Read the model definition and answer for the solid it produces. Units are mm, in the model's axes. A direction names the side the tool comes from. Give positions to 0.01 mm unless a question says otherwise; leave off trailing zeros. Write each loop counter-clockwise with the first axis right and the second up, starting at its lowest first coordinate (ties: lowest second). Pieces come first, ordered by that corner, then holes. Notation, with made-up numbers: (29.25, -19.75) - (52.25, -19.75) arc R8 cw to (52.25, -9.75) - close; hole circle Ø9 at (-30.75, -13.75). An arc over 180 degrees is marked (long way). Answer as CSV lines item,"result".
```python
from build123d import *

# Parameters (mm, degrees)
RESSALTO_EXTRUS_O1_DEPTH = 5
FILETE1_R                = 5
ESBO_O3_R                = 1.5
CORTE_EXTRUS_O1_DEPTH    = 5


with BuildPart() as part:
    # Esboço1 → Ressalto-extrusão1 (new body)
    with BuildSketch(Plane(origin=(0, 0, 0), x_dir=(1, 0, 0), z_dir=(0, 1, 0))):
        with BuildLine():
            Line((81.90590785, -20.429188404), (85.90590785, -20.429188404))
            Line((85.90590785, -20.429188404), (85.90590785, 4.570811596))
            ThreePointArc((85.90590785, 4.570811596), (84.441441756, 8.106345502), (80.90590785, 9.570811596))
            Line((80.90590785, 9.570811596), (-32.09409215, 9.570811596))
            ThreePointArc((-32.09409215, 9.570811596), (-35.629626056, 8.106345502), (-37.09409215, 4.570811596))
            Line((-37.09409215, 4.570811596), (-37.09409215, -20.429188404))
            Line((-37.09409215, -20.429188404), (-33.09409215, -20.429188404))
            Line((-33.09409215, -20.429188404), (-33.09409215, -75.429188404))
            Line((-33.09409215, -75.429188404), (-37.09409215, -75.429188404))
            Line((-37.09409215, -75.429188404), (-37.09409215, -100.429188404))
            ThreePointArc((-37.09409215, -100.429188404), (-35.629626056, -103.96472231), (-32.09409215, -105.429188404))
            Line((-32.09409215, -105.429188404), (80.90590785, -105.429188404))
            ThreePointArc((80.90590785, -105.429188404), (84.441441756, -103.96472231), (85.90590785, -100.429188404))
            Line((85.90590785, -100.429188404), (85.90590785, -75.429188404))
            Line((85.90590785, -75.429188404), (81.90590785, -75.429188404))
            Line((81.90590785, -75.429188404), (81.90590785, -20.429188404))
        make_face()
    extrude(amount=RESSALTO_EXTRUS_O1_DEPTH)

    # Filete1
    # the kernel refuses this fillet: 5 mm, written as the material it takes off along each edge
    with BuildSketch(Plane(origin=(-37.09409215, -12.247448714, 75.429188404), x_dir=(1.0, 0, 1.5738521597081158e-12), z_dir=(0, 1, 0)), Plane(origin=(85.90590785, -12.247448714, 20.429188404), x_dir=(-1.0, 0, -1.5685230891899197e-12), z_dir=(0, 1, 0))) as filete1_piece_1:
        with BuildLine():
            CenterArc((5, -4.898979486), FILETE1_R, 101.536959033, 78.463040967)
            Line((0, -4.898979486), (-0.1, -4.898979486))
            Line((-0.1, -4.898979486), (-0.1, 0))
            Line((-0.1, 0), (0, 0.1))
            ThreePointArc((0, 0.1), (2, 0.1), (3.98, 0.09797959))
            Line((3.98, 0.09797959), (4, 0))
        make_face()
    extrude(amount=29.494897428, mode=Mode.SUBTRACT)
    with BuildSketch(Plane(origin=(-37.09409215, -12.247448714, 20.429188404), x_dir=(0, 0, -1), z_dir=(0, 1, 0)), Plane(origin=(85.90590785, -12.247448714, 75.429188404), x_dir=(0, 0, 1), z_dir=(0, 1, 0))) as filete1_piece_2:
        with BuildLine():
            CenterArc((4.898979486, -5), FILETE1_R, 90, 78.463040967)
            Line((0, -4), (-0.09797959, -3.98))
            ThreePointArc((-0.09797959, -3.98), (-0.1, -2), (-0.1, 0))
            Line((-0.1, 0), (0, 0.1))
            Line((0, 0.1), (4.898979486, 0.1))
            Line((4.898979486, 0.1), (4.898979486, 0))
        make_face()
    extrude(amount=29.494897428, mode=Mode.SUBTRACT)

    # Esboço3 → Corte-extrusão1 (cut)
    with BuildSketch(Plane.XZ):
        with Locations(Location((-27.09409215, 5.429188404, 0), (0, 0, 270))):
            Circle(ESBO_O3_R)
        with Locations(Location((75.90590785, 5.429188404, 0), (0, 0, 270))):
            Circle(ESBO_O3_R)
        with Locations(Location((75.90590785, 90.429188404, 0), (0, 0, 90))):
            Circle(ESBO_O3_R)
        with Locations(Location((-27.09409215, 90.429188404, 0), (0, 0, 90))):
            Circle(ESBO_O3_R)
        with BuildLine():
            Line((35.90590785, 84.429188404), (35.90590785, 96.429188404))
            ThreePointArc((35.90590785, 96.429188404), (35.320121412, 97.843401966), (33.90590785, 98.429188404))
            Line((33.90590785, 98.429188404), (31.90590785, 98.429188404))
            ThreePointArc((31.90590785, 98.429188404), (30.491694287, 97.843401966), (29.90590785, 96.429188404))
            Line((29.90590785, 96.429188404), (29.90590785, 84.429188404))
            ThreePointArc((29.90590785, 84.429188404), (30.491694287, 83.014974841), (31.90590785, 82.429188404))
            Line((31.90590785, 82.429188404), (33.90590785, 82.429188404))
            ThreePointArc((33.90590785, 82.429188404), (35.320121412, 83.014974841), (35.90590785, 84.429188404))
        make_face()
        with BuildLine():
            Line((14.90590785, 13.429188404), (16.90590785, 13.429188404))
            ThreePointArc((16.90590785, 13.429188404), (18.320121412, 12.843401966), (18.90590785, 11.429188404))
            Line((18.90590785, 11.429188404), (18.90590785, -0.570811596))
            ThreePointArc((18.90590785, -0.570811596), (18.320121412, -1.985025159), (16.90590785, -2.570811596))
            Line((16.90590785, -2.570811596), (14.90590785, -2.570811596))
            ThreePointArc((14.90590785, -2.570811596), (13.491694287, -1.985025159), (12.90590785, -0.570811596))
            Line((12.90590785, -0.570811596), (12.90590785, 11.429188404))
            ThreePointArc((12.90590785, 11.429188404), (13.491694287, 12.843401966), (14.90590785, 13.429188404))
        make_face()
        with BuildLine():
            Line((23.40590785, 13.429188404), (25.40590785, 13.429188404))
            ThreePointArc((25.40590785, 13.429188404), (26.820121412, 12.843401966), (27.40590785, 11.429188404))
            Line((27.40590785, 11.429188404), (27.40590785, -0.570811596))
            ThreePointArc((27.40590785, -0.570811596), (26.820121412, -1.985025159), (25.40590785, -2.570811596))
            Line((25.40590785, -2.570811596), (23.40590785, -2.570811596))
            ThreePointArc((23.40590785, -2.570811596), (21.991694287, -1.985025159), (21.40590785, -0.570811596))
            Line((21.40590785, -0.570811596), (21.40590785, 11.429188404))
            ThreePointArc((21.40590785, 11.429188404), (21.991694287, 12.843401966), (23.40590785, 13.429188404))
        make_face()
        with BuildLine():
            Line((31.90590785, 13.429188404), (33.90590785, 13.429188404))
            ThreePointArc((33.90590785, 13.429188404), (35.320121412, 12.843401966), (35.90590785, 11.429188404))
            Line((35.90590785, 11.429188404), (35.90590785, -0.570811596))
            ThreePointArc((35.90590785, -0.570811596), (35.320121412, -1.985025159), (33.90590785, -2.570811596))
            Line((33.90590785, -2.570811596), (31.90590785, -2.570811596))
            ThreePointArc((31.90590785, -2.570811596), (30.491694287, -1.985025159), (29.90590785, -0.570811596))
            Line((29.90590785, -0.570811596), (29.90590785, 11.429188404))
            ThreePointArc((29.90590785, 11.429188404), (30.491694287, 12.843401966), (31.90590785, 13.429188404))
        make_face()
        with BuildLine():
            Line((27.40590785, 84.429188404), (27.40590785, 96.429188404))
            ThreePointArc((27.40590785, 96.429188404), (26.820121412, 97.843401966), (25.40590785, 98.429188404))
            Line((25.40590785, 98.429188404), (23.40590785, 98.429188404))
            ThreePointArc((23.40590785, 98.429188404), (21.991694287, 97.843401966), (21.40590785, 96.429188404))
            Line((21.40590785, 96.429188404), (21.40590785, 84.429188404))
            ThreePointArc((21.40590785, 84.429188404), (21.991694287, 83.014974841), (23.40590785, 82.429188404))
            Line((23.40590785, 82.429188404), (25.40590785, 82.429188404))
            ThreePointArc((25.40590785, 82.429188404), (26.820121412, 83.014974841), (27.40590785, 84.429188404))
        make_face()
        with BuildLine():
            Line((18.90590785, 84.429188404), (18.90590785, 96.429188404))
            ThreePointArc((18.90590785, 96.429188404), (18.320121412, 97.843401966), (16.90590785, 98.429188404))
            Line((16.90590785, 98.429188404), (14.90590785, 98.429188404))
            ThreePointArc((14.90590785, 98.429188404), (13.491694287, 97.843401966), (12.90590785, 96.429188404))
            Line((12.90590785, 96.429188404), (12.90590785, 84.429188404))
            ThreePointArc((12.90590785, 84.429188404), (13.491694287, 83.014974841), (14.90590785, 82.429188404))
            Line((14.90590785, 82.429188404), (16.90590785, 82.429188404))
            ThreePointArc((16.90590785, 82.429188404), (18.320121412, 83.014974841), (18.90590785, 84.429188404))
        make_face()
    extrude(amount=-CORTE_EXTRUS_O1_DEPTH, mode=Mode.SUBTRACT)


solid = part.part
```
(1) A cutting plane is placed at B-B (y = 0.85). Count the separate pieces of the cut face and the enclosed holes in it, and give its area (3 significant figures).
Worked out:
separate pieces,"1"
enclosed holes,"10"
area,"13,100 mm^2"
(2) The mould has two halves that part along Z. Classify faces 1 (the cylindrical face through (84.75, 2.46, 18.73)), 2 (the cylindrical face through (84.402, 2.465, 104.003)), 3 (the flat face through (85.906, 2, 91)): +Z half, -Z half, draft (parallel to the pull), parting line (faces both ways), or undercut.
Worked out:
face 1,"undercut"
face 2,"+Z half"
face 3,"draft"
(3) Find the intervals of material crossed by L1, parallel to X at y = 2.6, z = 10; L2, parallel to X at y = 4.05, z = 90.5; L3, parallel to Z at x = 77, y = 1.2, in increasing order.
Worked out:
L1,"x = -37.09 to 12.91, 18.91 to 21.41, 27.41 to 29.91, 35.91 to 85.91"
L2,"x = -37.09 to -28.59, -25.6 to 12.91, 18.91 to 21.41, 27.41 to 29.91, 35.91 to 74.41, 77.4 to 85.91"
L3,"z = -9.57 to 4.4, 6.46 to 89.4, 91.46 to 105.43"
(4) A cutting plane is placed at A-A (z = 29.5). Write down the section's boundary in (x, y).
Worked out:
outline,"(-33.09, 0) - (81.91, 0) - (81.91, 5) - (-33.09, 5) - close"
(5) For faces 4 (the flat face through (29.906, 2, 5)), 5 (the cylindrical face through (-35.94, 2.46, 77.13)), 6 (the flat face through (81.906, 2, 48)), determine the directions among +Z, -Z, +X, -X, +Y, -Y from which every point of the face is accessible in a straight line to the end or side of a thin tool.
Worked out:
face 4,"+Y, -Y"
face 5,"-X, +Y, -Y"
face 6,"+X, +Y, -Y"
(6) Each of these flat-tipped pins is pushed along its axis until it touches: P1, Ø5, axis at x = -27.09, z = 5.43, coming from the +Y side; P2, Ø1, axis at y = 3, z = 25.5, coming from the +X side. Where does it stop, or does it pass through?
Worked out:
P1,"stops at y = 5"
P2,"stops at x = 81.91"
